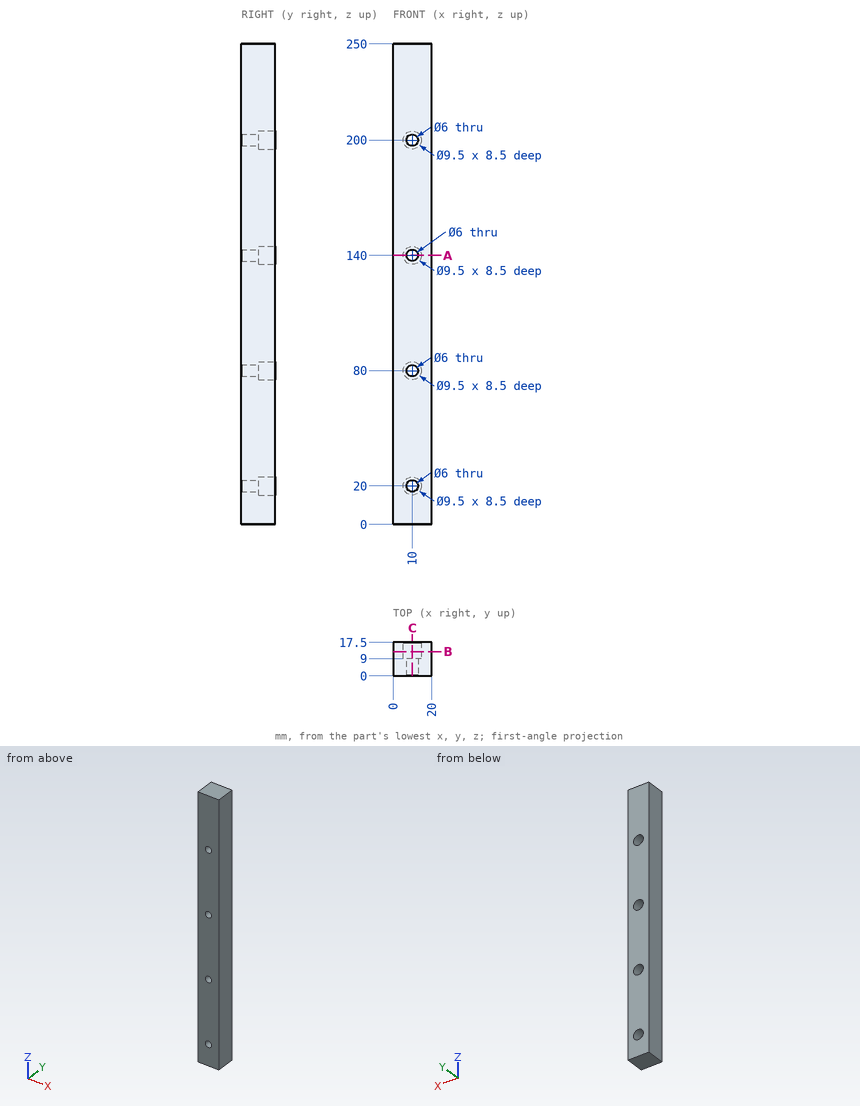
Design review of the part shown in the three views and the two pictorial views. Dimensions are in mm from the part's minimum x, y and z. Coordinates: 2 decimals unless noted, no trailing zeros. Order: outer loops, then holes, each group sorted by start corner. A loop starts at its lowest first (then second) coordinate and runs counter-clockwise, first axis right, second up. Notation, with made-up numbers: (28.25, 5.25) -> (71.25, 5.25) arc R17 ccw to (71.25, 35.25) -> close; hole circle Ø10 at (4, -28). An arc over 180 degrees is marked (long way). Use one line per item in the form item = value. Start each with the question number.
(1) Add section B-B on y = 12.75. State the section outline as (x, z) points.
(2) Insertion check: pin 1 (7.5 mm diameter, centred on x = 10, z = 20, fed in from +Y). The pin has a flat end and moves straight along its axis. Give the tip position at first contact, or say it passes through.
(3) For probe 1 along Z at (x, y) = (10, 2.25); probe 2 along Z at (x, y) = (10, 13); probe 3 along X at (y, z) = (11, 200), list the stretches that pass through material, from the lowest coordinate up.
(4) Add section A-A on z = 140. State the section outline as (x, y) points.
(5) Add section C-C on x = 10. Give the number of separate pieces and of enclosed holes in the cut face, plus the area to 3 significant figures.
Answer block:
q1.outline = (0, 0) -> (20, 0) -> (20, 250) -> (0, 250) -> close; hole circle Ø9.5 at (10, 20); hole circle Ø9.5 at (10, 80); hole circle Ø9.5 at (10, 140); hole circle Ø9.5 at (10, 200)
q2.pin_1 = 9
q3.probe_1 = 0 to 17, 23 to 77, 83 to 137, 143 to 197, 203 to 250
q3.probe_2 = 0 to 15.25, 24.75 to 75.25, 84.75 to 135.25, 144.75 to 195.25, 204.75 to 250
q3.probe_3 = 0 to 5.25, 14.75 to 20
q4.outline = (0, 0) -> (7, 0) -> (7, 9) -> (5.25, 9) -> (5.25, 17.5) -> (0, 17.5) -> close; (13, 0) -> (20, 0) -> (20, 17.5) -> (14.75, 17.5) -> (14.75, 9) -> (13, 9) -> close
q5.separate_pieces = 5
q5.enclosed_holes = 0
q5.area = 3,840 mm²
